Geometry: final body of the model. Coordinates: model frame, mm. Round coordinates to 2 decimals unless told otherwise and drop trailing zeros. Loops run counter-clockwise (first coordinate to the right, second up) from the corner with the lowest first, then second, coordinate; pieces in that order, holes last. Notation, with made-up numbers: M -6.5,32 L -1.5,32 A18 cw -1.5,56 Z; hole C 45,73.5 d4. An arc over 180 degrees is marked long. Return JSON: item names as keys, results as strings.
from build123d import *

# Parameters (mm, degrees)
F0_W     = 800
F0_H     = 1800
F1_DEPTH = 200
F3_W     = 50
F3_H     = 1600
F4_DEPTH = 100
F5_W     = 100
F5_H     = 60
F6_DEPTH = 800


with BuildPart() as f1:
    # F0 (on Front) → F1 (new body)
    with BuildSketch(Plane.XZ):
        with Locations((400, 900)):
            Rectangle(F0_W, F0_H)
    extrude(amount=F1_DEPTH)

    # F3 (on face) → F4 (cut)
    with BuildSketch(Plane.XZ.offset(200)):
        with Locations((75, 900)):
            Rectangle(F3_W, F3_H)
        with Locations((725, 900)):
            Rectangle(F3_W, F3_H)
    extrude(amount=-F4_DEPTH, mode=Mode.SUBTRACT)

    # F5 (on face) → F6 (join)
    with BuildSketch(Plane.XZ.offset(200)):
        with Locations((50, 30)):
            Rectangle(F5_W, F5_H)
        with Locations((750, 30)):
            Rectangle(F5_W, F5_H)
    extrude(amount=F6_DEPTH)


solid = f1.part
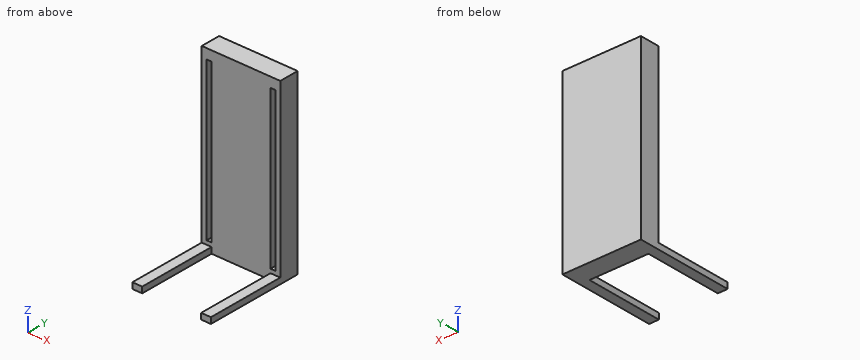
Q1. Section query B-B (x = 73). Output: boundary loops of the cut face in (y, z).
Determined:
{"outline": "M -1000,0 L 0,0 L 0,1800 L -200,1800 L -200,1700 L -100,1700 L -100,100 L -200,100 L -200,60 L -1000,60 Z"}
Q2. Section query D-D (x = 646). Output: boundary loops of the cut face in (y, z).
Determined:
{"outline": "M -200,0 L 0,0 L 0,1800 L -200,1800 Z"}
Q3. Pin query (flat end, axial travel): pin 1 (1 mm diameter, centred on x = 288, z = 1056.5, fed in from -Y); pin 2 (15 mm diameter, centred on x = 714, z = 735, fed in from -Y). Return the tip coordinate at first contact, or that it passes through.
Determined:
{"pin 1": "stops at y = -200", "pin 2": "stops at y = -100"}
Q4. Section query C-C (z = 1507). Output: boundary loops of the cut face in (x, y), plus the area to 3 significant figures.
Determined:
{"outline": "M 0,-200 L 50,-200 L 50,-100 L 100,-100 L 100,-200 L 700,-200 L 700,-100 L 750,-100 L 750,-200 L 800,-200 L 800,0 L 0,0 Z", "area": "150,000 mm^2"}
Q5. Material intervals for L1, parallel to X at y = -107.5, z = 104.5; L2, parallel to Y at x = 481.5, z = 1324; L3, parallel to Y at x = 91, z = 274, sorted ascending.
Determined:
{"L1": "x = 0 to 50, 100 to 700, 750 to 800", "L2": "y = -200 to 0", "L3": "y = -100 to 0"}
Q6. Section query A-A (y = -653.5). Output: boundary loops of the cut face in (x, z).
Determined:
{"outline": "M 0,0 L 100,0 L 100,60 L 0,60 Z; M 700,0 L 800,0 L 800,60 L 700,60 Z"}
